The model under review builds one solid part; all positions refer to its coordinate system, in mm. Face numbers are marked on the shaded views. Give positions to 0.01 mm unless a question says otherwise; leave off trailing zeros. Order: outer loops, then holes, each group sorted by start corner. A loop starts at its lowest first (then second) coordinate and runs counter-clockwise, first axis right, second up.
```python
from build123d import *

# Parameters (mm, degrees)
F0_W        = 101.5806943178
F0_H        = 48.01966995
F1_DEPTH    = 105.5511329323
F2_R        = 29.2525430431
F3_T1_DEPTH = 554.2240944956
F4_SIZE     = 5.08
F5_T2_ANGLE = 31.2878347999
F7_D        = 6.35
F9_ANGLE    = 180


# Not quite as in the source:
# - a fillet or chamfer that OpenCascade refuses, or shapes differently, is made with other operations: its cross-section is extruded or revolved along the edge and cut away or added


with BuildPart() as f1:
    # F0 (on Top) → F1 (new body)
    with BuildSketch(Plane.XY):
        with Locations((9.8017528653, 24.009834975)):
            Rectangle(F0_W, F0_H)
    extrude(amount=F1_DEPTH)

    # F2
    f2_edges = [f1.edges().sort_by_distance(p)[0] for p in [
        (9.801753, 0, 105.551133),
    ]]
    fillet(f2_edges, radius=F2_R)

    # F3: fillet of radius 227.7292364389 on 1 edges, made by hand

    # F3_s2 → F3_t1 (cut)
    with BuildSketch(Plane.YZ.offset(-267.3102943825)):
        with BuildLine():
            ThreePointArc((29.2525430431, 105.5511329323), (43.2785349621, 61.2491955933), (48.01966995, 15.0224528968))
            Line((48.01966995, 15.0224528968), (48.01966995, 105.5511329323))
            Line((48.01966995, 105.5511329323), (29.2525430431, 105.5511329323))
        make_face()
    extrude(amount=F3_T1_DEPTH, mode=Mode.SUBTRACT)

    # F4
    f4_edges = [f1.edges().sort_by_distance(p)[0] for p in [
        (9.801753, 0, 0),
    ]]
    chamfer(f4_edges, length=F4_SIZE)

    # F5: chamfer of 5.08 on 1 edges, made by hand

    # F5_s1 → F5_t2 (revolve, cut)
    with BuildSketch(Plane(origin=(0, -44.077363084, 85.1947407747), x_dir=(1, 0, 0), z_dir=(0, -0.4595143579, 0.8881703411))):
        with BuildLine():
            Line((61.6697307588, 68.8619315298), (54.4344692897, 76.0971929988))
            Line((54.4344692897, 76.0971929988), (54.4344692897, 76.8591929988))
            ThreePointArc((54.4344692897, 76.8591929988), (57.513284657, 75.7815622643), (60.5921000242, 75.7815622643))
            Line((60.5921000242, 75.7815622643), (61.3541000242, 75.0195622643))
            ThreePointArc((61.3541000242, 75.0195622643), (61.3541000242, 71.9407468971), (62.4317307588, 68.8619315298))
            Line((62.4317307588, 68.8619315298), (61.6697307588, 68.8619315298))
        make_face()
    revolve(axis=Axis((60.5921000242, -179.7095664878, 15.022452897), (-1, 0, 0)), revolution_arc=F5_T2_ANGLE, mode=Mode.SUBTRACT)

    # F7 (through all)
    with Locations(Plane.XZ):
        with Locations((0, 37.8390811384)):
            Hole(F7_D / 2)

    # F8: F1 across plane


with BuildPart() as f1_1:
    add(f1.part)
    add(f1.part.mirror(Plane.XZ))

    # F8_face (on face) → F9 (revolve)
    with BuildSketch(Plane(origin=(60.5921000242, 0, 46.1455237947), x_dir=(0, 1, 0), z_dir=(1, 0, 0))):
        with BuildLine():
            Line((0, -41.0655237947), (5.08, -46.1455237947))
            Line((5.08, -46.1455237947), (42.432298984, -46.1455237947))
            ThreePointArc((42.432298984, -46.1455237947), (39.5623129602, 7.5101449883), (23.9216912378, 58.9157727391))
            ThreePointArc((23.9216912378, 58.9157727391), (6.7619645003, 48.8582833159), (0, 30.1530660945))
            ThreePointArc((0, 30.1530660945), (-6.7619645003, 48.8582833159), (-23.9216912378, 58.9157727391))
            ThreePointArc((-23.9216912378, 58.9157727391), (-39.5623129602, 7.5101449883), (-42.432298984, -46.1455237947))
            Line((-42.432298984, -46.1455237947), (-5.08, -46.1455237947))
            Line((-5.08, -46.1455237947), (0, -41.0655237947))
        make_face()
    revolve(axis=Axis((60.5921000242, -23.756149492, 0), (0, 1, 0)), revolution_arc=F9_ANGLE)

    # F10: F1 across face


with BuildPart() as f1_2:
    add(f1_1.part)
    add(f1_1.part.mirror(Plane(origin=(9.6264102551, 26.4795740308, 0), x_dir=(1, 0, 0), z_dir=(0, 0, -1))))

    # F11: F1 across face


with BuildPart() as f1_3:
    add(f1_2.part)
    add(f1_2.part.mirror(Plane(origin=(-40.9885942936, 0, 0), x_dir=(0, -1, 0), z_dir=(-1, 0, 0))))


solid = f1_3.part
```
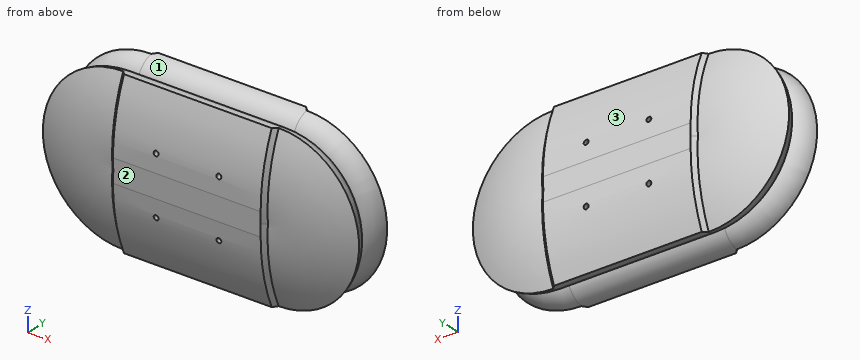
1. Draft analysis for pull direction Y (two halves, no side actions). For the marked faces 1, 2 and 3, state which applies: pulls with the +Y half, pulls with the -Y half, needs draft (parallel to the pull), parting line crosses it, or undercut.
2. Insertion check: pin 1 (5 mm diameter, centred on y = 21.5, z = 51.5, fed in from +X); pin 2 (1 mm diameter, centred on x = -77, z = -18.5, fed in from -Y); pin 3 (2 mm diameter, centred on y = -22, z = -39, fed in from -X). Each pin has a flat end and moves straight along its axis. Give the tip position at first contact, or say it passes through.
3. Take a section at A-A (x = -8.5). Write out the cut boundary in (y, z), and give its area (3 significant figures).
4. To check wall thickness, follow line 1 (Z direction, x = 0, y = -8); line 2 (Y direction, x = -20, z = 96); line 3 (Y direction, x = -76, z = -94.5). State the ranges of each line that lie inside material, in increasing order.
Answer:
1. face 1: undercut
1. face 2: pulls with the -Y half
1. face 3: pulls with the +Y half
2. pin 1: stops at x = 153.08
2. pin 2: stops at y = -48
2. pin 3: stops at x = -240.14
3. outline: (-48.02, -15.02) arc R227.73 ccw to (-29.25, -105.55) arc R29.25 ccw to (0, -76.3) arc R29.25 ccw to (29.25, -105.55) arc R227.73 ccw to (48.02, -15.02) - (48.02, 15.02) arc R227.73 ccw to (29.25, 105.55) arc R29.25 ccw to (0, 76.3) arc R29.25 ccw to (-29.25, 105.55) arc R227.73 ccw to (-48.02, 15.02) - close; hole (-5.08, 0) - (0, -5.08) - (5.08, 0) - (0, 5.08) - close
3. area: 17,300 mm2
4. line 1: z = -96.4 to -41.01, -34.66 to 34.66, 41.01 to 96.4
4. line 2: y = -33.14 to -7.63, 7.63 to 33.14
4. line 3: y = -33.7 to -6.35, 6.35 to 33.7
